from build123d import *

# Parameters (mm, degrees)
SKETCH1_W           = 25.4
SKETCH1_H           = 25.4
SKETCH1_W_2         = 22.9108
SKETCH1_H_2         = 22.9108
BOSS_EXTRUDE1_DEPTH = 210.82
SKETCH2_R           = 12.7
CUT_EXTRUDE1_DEPTH  = 210.82
SKETCH3_R           = 3.175
CUT_EXTRUDE2_DEPTH  = 1.2446


with BuildPart() as part:
    # Sketch1 → Boss-Extrude1 (new body)
    with BuildSketch(Plane(origin=(0, 0, 0), x_dir=(1, 0, 0), z_dir=(0, 1, 0))):
        Rectangle(SKETCH1_W, SKETCH1_H)
        Rectangle(SKETCH1_W_2, SKETCH1_H_2, mode=Mode.SUBTRACT)
    extrude(amount=BOSS_EXTRUDE1_DEPTH)

    # Sketch2 → Cut-Extrude1 (cut)
    with BuildSketch(Plane(origin=(12.7, 0, 0), x_dir=(0, 0, -1), z_dir=(1, 0, 0))):
        with Locations((-1.2446, 147.32)):
            Circle(SKETCH2_R)
        with Locations((-13.9446, 13.97)):
            Circle(SKETCH2_R)
    extrude(amount=-CUT_EXTRUDE1_DEPTH, mode=Mode.SUBTRACT)

    # Sketch3 → Cut-Extrude2 (cut)
    with BuildSketch(Plane(origin=(0, 0, -12.7), x_dir=(-1, 0, 0), z_dir=(0, 0, -1))):
        with Locations((0, 197.1675)):
            Circle(SKETCH3_R)
        with Locations((0, 14.2875)):
            Circle(SKETCH3_R)
    extrude(amount=-CUT_EXTRUDE2_DEPTH, mode=Mode.SUBTRACT)


solid = part.part
Geometry: final body of the model. Coordinates: model frame, mm. A direction names the side the tool comes from. Round coordinates to 2 decimals unless told otherwise and drop trailing zeros. Loops run counter-clockwise (first coordinate to the right, second up) from the corner with the lowest first, then second, coordinate; pieces in that order, holes last.
Q1. Section D-D on z = 6.5. Return loops of the section in (x, y), plus the area to 3 significant figures.
Q2. Access query for faces 5 (the cylindrical face through (0.413, 200.315, -12.086)), 6 (the flat face through (12.7, 104, 0)), 7 (the flat face through (-11.455, 73, 0)). Directions: +Z, -Z, +X, -X, +Y, -Y. A direction counts if a zero-diameter tool reaches every point of the face in a straight line with its end or side. Return the directions, or none.
Q3. Pull-direction query (Y, two-part tool) for faces 1 (the flat face through (-1, 210.82, 12)), 2 (the flat face through (-1, 0, 12)), 3 (the flat face through (11.455, 73, 0)), 4 (the cylindrical face through (0.69, 11.19, -12.09)); classes: released by +Y, released by -Y, zero draft, split by the parting line, or undercut.
Q4. Pin query (flat end, axial travel): P1, Ø3, axis at x = 5, z = -10, coming from the +Y side; P2, Ø5.5, axis at x = 0, y = 197.17, coming from the -Z side. Return the tip coordinate at first contact, or that it passes through.
Q5. Material intervals for L1, parallel to Y at x = 0, z = -11.95; L2, parallel to X at y = 23.5, z = -5, sorted ascending.
Q6. Section B-B on y = 178. Return loops of the section in (x, z).
Q7. Section C-C on z = -3.25. Return loops of the section in (x, y).
Q8. Section A-A on x = -7.25. Return loops of the section in (y, z), plus the area to 3 significant figures.
Evaluation:
1. outline: (-12.7, 0) - (-11.46, 0) - (-11.46, 3.68) - (-12.7, 3.68) - close; (-12.7, 24.26) - (-11.46, 24.26) - (-11.46, 135.76) - (-12.7, 135.76) - close; (-12.7, 158.88) - (-11.46, 158.88) - (-11.46, 210.82) - (-12.7, 210.82) - close; (11.46, 0) - (12.7, 0) - (12.7, 3.68) - (11.46, 3.68) - close; (11.46, 24.26) - (12.7, 24.26) - (12.7, 135.76) - (11.46, 135.76) - close; (11.46, 158.88) - (12.7, 158.88) - (12.7, 210.82) - (11.46, 210.82) - close
1. area: 416 mm2
2. face 5: -Z
2. face 6: +Z, -Z, +X, +Y, -Y
2. face 7: +Y, -Y
3. face 1: released by +Y
3. face 2: released by -Y
3. face 3: zero draft
3. face 4: undercut
4. P1: stops at y = 210.82
4. P2: stops at z = 11.46
5. L1: y = 0 to 11.11, 17.46 to 193.99, 200.34 to 210.82
5. L2: x = -12.7 to -11.46, 11.46 to 12.7
6. outline: (-12.7, -12.7) - (12.7, -12.7) - (12.7, 12.7) - (-12.7, 12.7) - close; hole (-11.46, -11.46) - (11.46, -11.46) - (11.46, 11.46) - (-11.46, 11.46) - close
7. outline: (-12.7, 0) - (-11.46, 0) - (-11.46, 135.44) - (-12.7, 135.44) - close; (-12.7, 159.2) - (-11.46, 159.2) - (-11.46, 210.82) - (-12.7, 210.82) - close; (11.46, 0) - (12.7, 0) - (12.7, 135.44) - (11.46, 135.44) - close; (11.46, 159.2) - (12.7, 159.2) - (12.7, 210.82) - (11.46, 210.82) - close
8. outline: (0, -12.7) - (210.82, -12.7) - (210.82, -11.46) - (0, -11.46) - close; (0, 11.46) - (1.52, 11.46) arc R12.7 cw to (1.33, 12.7) - (0, 12.7) - close; (26.42, 11.46) - (139.77, 11.46) arc R12.7 cw to (141.84, 12.7) - (26.61, 12.7) arc R12.7 cw to start; (152.8, 12.7) arc R12.7 cw to (154.87, 11.46) - (210.82, 11.46) - (210.82, 12.7) - close
8. area: 477 mm2
